Geometry check sheet. Reference: the model listing, model coordinates, mm. Face numbers are marked on the shaded views. A direction names the side the tool comes from. Round coordinates to 2 decimals unless told otherwise and drop trailing zeros. Order: outer loops, then holes, each group sorted by start corner. A loop starts at its lowest first (then second) coordinate and runs counter-clockwise, first axis right, second up. Notation, with made-up numbers: (54.25, -31) - (61.25, -31) arc R23 cw to (61.25, -5) - close; hole circle Ø1 at (69.5, 40.25). An arc over 180 degrees is marked (long way). Return JSON: item names as keys, results as strings. Group by question number.
Q1. Sectioned sample at B-B, the plane z = 36. Record the cut outline in (x, y), then the cut area to 3 significant figures.
Q2. Tool access check on the marked faces 5 and 6. Record the directions out of +Z, -Z, +X, -X, +Y, -Y that give a thin tool (end or side, any length) a straight path to the whole face; none if there is none.
Q3. Draft check along Y on the marked faces 1, 2, 3 and 4. Enter one of: pulls with the +Y half, pulls with the -Y half, needs draft (parallel to the pull), parting line crosses it, or undercut.
Q4. Sectioned sample at C-C, the plane x = -24.3. Record the cut outline in (y, z), then the cut area to 3 significant figures.
Q5. Sectioned sample at A-A, the plane x = -11.6. Record the cut outline in (y, z), then the cut area to 3 significant figures.
Q6. Sectioned sample at D-D, the plane y = 32. Record the cut outline in (x, z).
Q7. Gauge pin test, flat ends, axial feed: pin 1 Ø5 at (x, z) = (-12, 25) entering from +Y; pin 2 Ø9 at (x, y) = (-24.3, 34) entering from -Z; pin 3 Ø4 at (x, y) = (-26.5, 35.5) entering from +Z; pin 4 Ø3.5 at (y, z) = (37, 2.5) entering from +X. Record the tip position at first contact, or that the pin passes through.
Q8. Material ranges on line 1 along Y through (x, z) = (-24.3, 0.95); line 2 along Y through (x, z) = (-11.6, 25.5); line 3 along X through (y, z) = (12, 26), recorded low to high.
```python
from build123d import *

# Parameters (mm, degrees)
SKETCH1_R           = 2.75
BOSS_EXTRUDE1_DEPTH = 8
SKETCH2_W           = 43.1
SKETCH2_H           = 25
SKETCH2_R           = 2.75
BOSS_EXTRUDE2_DEPTH = 31
CHAMFER1_SIZE       = 6.5
FILLET1_R           = 5
CUT_EXTRUDE1_DEPTH  = 4
FILLET2_R           = 3


with BuildPart() as part:
    # Sketch1 → Boss-Extrude1 (new body)
    with BuildSketch(Plane.XY):
        Polygon((0, 0), (-43.1, 0), (-43.1, 42), (-11, 42), (-11, 35.920164834), (0, 25), align=None)
        with Locations((-11.6, 12.7)):
            Circle(SKETCH1_R, mode=Mode.SUBTRACT)
        with Locations((-24.3, 12.7)):
            Circle(SKETCH1_R, mode=Mode.SUBTRACT)
        with Locations((-37, 12.7)):
            Circle(SKETCH1_R, mode=Mode.SUBTRACT)
        with Locations((-24.3, 34)):
            Circle(SKETCH1_R, mode=Mode.SUBTRACT)
    extrude(amount=BOSS_EXTRUDE1_DEPTH)

    # Sketch2 → Boss-Extrude2 (add)
    with BuildSketch(Plane.XY.offset(8)):
        with Locations((-21.55, 12.5)):
            Rectangle(SKETCH2_W, SKETCH2_H)
        with Locations((-11.6, 12.7)):
            Circle(SKETCH2_R, mode=Mode.SUBTRACT)
        with Locations((-24.3, 12.7)):
            Circle(SKETCH2_R, mode=Mode.SUBTRACT)
        with Locations((-37, 12.7)):
            Circle(SKETCH2_R, mode=Mode.SUBTRACT)
    extrude(amount=BOSS_EXTRUDE2_DEPTH)

    # Chamfer1
    chamfer1_edges = [part.edges().sort_by_distance(p)[0] for p in [
        (-43.1, 0, 19.5),
        (-43.1, 25, 23.5),
    ]]
    chamfer(chamfer1_edges, length=CHAMFER1_SIZE)

    # Fillet1
    fillet1_edges = [part.edges().sort_by_distance(p)[0] for p in [
        (-18.3, 25, 8),
        (-39.85, 21.75, 8),
    ]]
    fillet(fillet1_edges, radius=FILLET1_R)

    # Sketch3 → Cut-Extrude1 (cut)
    with BuildSketch(Plane.XY.offset(8)):
        Polygon((-19.681197846, 34), (-21.990598923, 38), (-26.609401077, 38), (-28.918802154, 34), (-26.609401077, 30), (-21.990598923, 30), align=None)
    extrude(amount=-CUT_EXTRUDE1_DEPTH, mode=Mode.SUBTRACT)

    # Fillet2
    fillet2_edges = [part.edges().sort_by_distance(p)[0] for p in [
        (-43.1, 42, 4),
        (-11, 42, 4),
    ]]
    fillet(fillet2_edges, radius=FILLET2_R)


solid = part.part
```
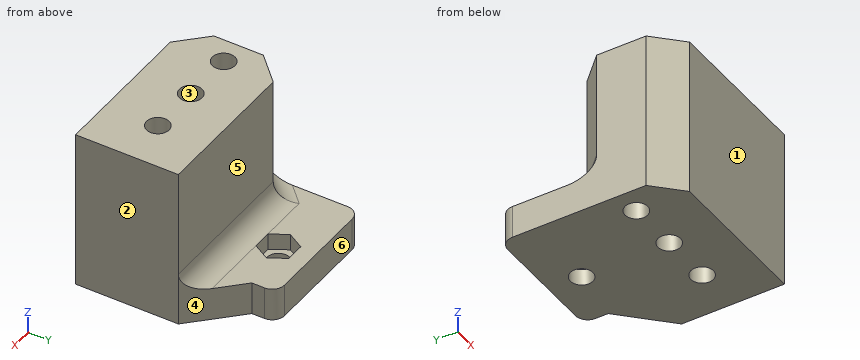
Reply:
{
 "1": {"outline": "(-43.1, 6.5) - (-36.6, 0) - (0, 0) - (0, 25) - (-36.6, 25) - (-43.1, 18.5) - close; hole circle Ø5.5 at (-37, 12.7); hole circle Ø5.5 at (-24.3, 12.7); hole circle Ø5.5 at (-11.6, 12.7)", "area": "964 mm^2"},
 "2": {"face 5": "+Z, +X, -X, +Y", "face 6": "+Z, -Z, +X, -X, +Y"},
 "3": {"face 1": "pulls with the -Y half", "face 2": "needs draft", "face 3": "undercut", "face 4": "pulls with the +Y half"},
 "4": {"outline": "(0, 0) - (9.95, 0) - (9.95, 39) - (0, 39) - close; (15.45, 0) - (31.25, 0) - (31.25, 4) - (30, 4) - (30, 8) arc R5 cw to (25, 13) - (25, 39) - (15.45, 39) - close; (36.75, 0) - (42, 0) - (42, 8) - (38, 8) - (38, 4) - (36.75, 4) - close", "area": "848 mm^2"},
 "5": {"outline": "(0, 0) - (9.95, 0) - (9.95, 39) - (0, 39) - close; (15.45, 0) - (40.8, 0) - (40.8, 8) - (30, 8) arc R5 cw to (25, 13) - (25, 39) - (15.45, 39) - close", "area": "892 mm^2"},
 "6": {"outline": "(-43.1, 0) - (-26.19, 0) - (-26.19, 4) - (-27.76, 4) - (-27.76, 8) - (-43.1, 8) - close; (-22.41, 0) - (-7.05, 0) - (-7.05, 8) - (-20.84, 8) - (-20.84, 4) - (-22.41, 4) - close"},
 "7": {"pin 1": "y = 25", "pin 2": "z = 0", "pin 3": "z = 8", "pin 4": "x = -10.32"},
 "8": {"line 1": "0 to 9.95, 15.45 to 31.25, 36.75 to 42", "line 2": "0 to 9.95, 15.45 to 25", "line 3": "-43.1 to -39.66, -34.34 to -26.96, -21.64 to -14.26, -8.94 to 0"}
}
